```python
from build123d import *

# Parameters (mm, degrees)
F0_R     = 11.0109
F1_DEPTH = 6.35


with BuildPart() as f1:
    # F0 (on Front) → F1 (new body)
    with BuildSketch(Plane.XZ):
        with BuildLine():
            ThreePointArc((-12.3733379796, 24.6062500399), (-0.0274921787, 17.4625264504), (12.3457542252, 24.5586851785))
            ThreePointArc((12.3457542252, 24.5586851785), (13.7935242005, 28.0255743558), (14.2875, 31.75))
            ThreePointArc((14.2875, 31.75), (-3.6978770846, 45.5506652491), (-12.3733379796, 24.6062500399))
        make_face()
        with Locations((0, 31.75)):
            Circle(F0_R, mode=Mode.SUBTRACT)
        with BuildLine():
            ThreePointArc((-12.3733379176, 7.1437500675), (-0.6313413892, 14.2735442095), (11.6942925407, 8.2082993502))
            ThreePointArc((11.6942925407, 8.2082993502), (9.9863540663, 16.4645214005), (12.3457542252, 24.5586851785))
            ThreePointArc((12.3457542252, 24.5586851785), (-0.0274921787, 17.4625264504), (-12.3733379796, 24.6062500399))
            ThreePointArc((-12.3733379796, 24.6062500399), (-10.6288268346, 20.3946275974), (-10.0338065702, 15.875))
            ThreePointArc((-10.0338065702, 15.875), (-10.6288268185, 11.3553724626), (-12.3733379176, 7.1437500675))
        make_face()
        with BuildLine():
            ThreePointArc((-0.0549843517, -14.2873941981), (10.0833294929, -10.1222093728), (14.2875, 0))
            ThreePointArc((14.2875, 0), (13.9564974416, 3.057586534), (12.9788266264, 5.9735011218))
            ThreePointArc((12.9788266264, 5.9735011218), (12.2952680668, 7.0671663883), (11.6942925407, 8.2082993502))
            ThreePointArc((11.6942925407, 8.2082993502), (-0.6313413892, 14.2735442095), (-12.3733379176, 7.1437500675))
            ThreePointArc((-12.3733379176, 7.1437500675), (-12.3870611826, -7.1199277742), (-0.0549843517, -14.2873941981))
        make_face()
        Circle(F0_R, mode=Mode.SUBTRACT)
        with BuildLine():
            ThreePointArc((-15.2451557121, -23.0185149788), (-8.8243212537, -16.6100235917), (-0.0549843517, -14.2873941981))
            ThreePointArc((-0.0549843517, -14.2873941981), (-12.3870611826, -7.1199277742), (-12.3733379176, 7.1437500675))
            ThreePointArc((-12.3733379176, 7.1437500675), (-18.7941724786, 0.7352586382), (-27.5635095047, -1.5873706872))
            ThreePointArc((-27.5635095047, -1.5873706872), (-17.4962843274, -5.7914353078), (-13.3309936151, -15.8747648862))
            ThreePointArc((-13.3309936151, -15.8747648862), (-13.8178283859, -19.5726420447), (-15.2451557121, -23.0185149788))
        make_face()
        with BuildLine():
            ThreePointArc((-27.5635095047, -1.5873706872), (-40.0055547448, -22.9946927523), (-15.2451557121, -23.0185149788))
            ThreePointArc((-15.2451557121, -23.0185149788), (-13.8178283859, -19.5726420447), (-13.3309936151, -15.8747648862))
            ThreePointArc((-13.3309936151, -15.8747648862), (-17.4962843274, -5.7914353078), (-27.5635095047, -1.5873706872))
        make_face()
        with Locations((-27.6184936151, -15.8747648862)):
            Circle(F0_R, mode=Mode.SUBTRACT)
        with BuildLine():
            ThreePointArc((12.9788266264, 5.9735011218), (13.9564974416, 3.057586534), (14.2875, 0))
            ThreePointArc((14.2875, 0), (10.0833294929, -10.1222093728), (-0.0549843517, -14.2873941981))
            ThreePointArc((-0.0549843517, -14.2873941981), (8.6671977023, -16.6605097019), (15.034271116, -23.0767791104))
            ThreePointArc((15.034271116, -23.0767791104), (15.0754403986, -8.8131539558), (27.4350094206, -1.693199528))
            ThreePointArc((27.4350094206, -1.693199528), (19.2533298904, 0.3420834154), (12.9788266264, 5.9735011218))
        make_face()
        with BuildLine():
            ThreePointArc((41.7225094331, -15.980699528), (37.5377975649, -5.8779113874), (27.4350094206, -1.693199528))
            ThreePointArc((27.4350094206, -1.693199528), (15.0754403986, -8.8131539558), (15.034271116, -23.0767791104))
            ThreePointArc((15.034271116, -23.0767791104), (31.1063244253, -29.7884546851), (41.7225094331, -15.980699528))
        make_face()
        with Locations((27.4350094331, -15.980699528)):
            Circle(F0_R, mode=Mode.SUBTRACT)
    extrude(amount=F1_DEPTH)


solid = f1.part
```
CAD build for the part. Positions are in the model's coordinates, mm. Round coordinates to 2 decimals unless told otherwise and drop trailing zeros. Loops run counter-clockwise (first coordinate to the right, second up) from the corner with the lowest first, then second, coordinate; pieces in that order, holes last. Notation, with made-up numbers: M -25.75,28.5 L 20.25,28.5 A21 ccw 20.25,35.5 Z; hole C -31,27.5 d10. An arc over 180 degrees is marked long. Use a Markdown table: item, result. Add a question column.
(1) Cut at A-A (x = 25). Give the cut face in (y, z).
(2) Flat gauge pins, fed straight in: pin 1 (1.5 mm diameter, centred on x = 13, y = -3, fed in from -Z); pin 2 (4 mm diameter, centred on x = -1.5, z = -10, fed in from +Y); pin 3 (3 mm diameter, centred on y = -3, z = -6, fed in from -X); pin 4 (1 mm diameter, centred on x = -32, y = -3, fed in from -Z). Where does each tip first touch, or does it go through?
(3) Drill centre lines: line 1 (Z direction, x = 0, y = -1.5); line 2 (Z direction, x = -6, y = -5); line 3 (X direction, y = -0.5, z = -8). Where is each one in solid material? Low to high.
(4) Cut at C-C (z = -24). Give the cut face in (x, y).
(5) Pull direction Z, two halves, no side cores. Call faces 1 (the face through (-40.21, -3.13, -22.63)), 2 (the face through (32.516, -3.131, -25.749)), 3 (the face through (0, -6.35, -12)): +Z half, -Z half, draft (parallel to the pull), parting line (faces both ways), or undercut.
(6) Cut at B-B (z = 33.5). Give the cut face in (x, y), and give its area (3 significant figures).
(7) Cut at D-D (y = -2.25). State how many separate pieces and enclosed holes the cut face has, and give its area (3 significant figures).
Geometry says:
| question | item | result |
|---|---|---|
| 1 | outline | M -6.35,-30.06 L 0,-30.06 L 0,-26.72 L -6.35,-26.72 Z; M -6.35,-5.24 L 0,-5.24 L 0,-1.52 L -6.35,-1.52 Z |
| 2 | pin 1 | stops at z = -21.14 |
| 2 | pin 2 | stops at y = 0 |
| 2 | pin 3 | stops at x = -39.19 |
| 2 | pin 4 | stops at z = -29.62 |
| 3 | line 1 | z = -14.29 to -11.01, 11.01 to 20.74, 42.76 to 46.04 |
| 3 | line 2 | z = -15.31 to -9.23, 9.23 to 22.52, 40.98 to 44.72 |
| 3 | line 3 | x = -39.54 to -35.31, -19.92 to -7.57, 7.57 to 19.85, 35.02 to 39.29 |
| 4 | outline | M -39.37,-6.35 L -35.05,-6.35 L -35.05,0 L -39.37,0 Z; M -20.19,-6.35 L -15.87,-6.35 L -15.87,0 L -20.19,0 Z; M 15.61,-6.35 L 19.89,-6.35 L 19.89,0 L 15.61,0 Z; M 34.98,-6.35 L 39.26,-6.35 L 39.26,0 L 34.98,0 Z |
| 5 | face 1 | parting line |
| 5 | face 2 | undercut |
| 5 | face 3 | draft |
| 6 | outline | M -14.18,-6.35 L -10.87,-6.35 L -10.87,0 L -14.18,0 Z; M 10.87,-6.35 L 14.18,-6.35 L 14.18,0 L 10.87,0 Z |
| 6 | area | 42.0 mm² |
| 7 | separate pieces | 1 |
| 7 | enclosed holes | 4 |
| 7 | area | 1,420 mm² |
